Part model, mm, in its own coordinate system. A direction names the side the tool comes from. Round coordinates to 2 decimals unless told otherwise and drop trailing zeros. Order: outer loops, then holes, each group sorted by start corner. A loop starts at its lowest first (then second) coordinate and runs counter-clockwise, first axis right, second up. Notation, with made-up numbers: (-0.75, 68.25) -> (44.25, 68.25) arc R31 ccw to (44.25, 95.25) -> close; hole circle Ø8 at (-10, 57.5). An arc over 180 degrees is marked (long way). Use CSV: the item, a comma, the result in double quotes.
```python
from build123d import *

# Parameters (mm, degrees)
SKETCH_R     = 2.5
PAD_DEPTH    = 2
PAD001_DEPTH = 5
SKETCH002_R  = 2.5
PAD002_DEPTH = 30
PAD003_DEPTH = 5
SKETCH004_R  = 2.5
PAD004_DEPTH = 3


with BuildPart() as part:
    # Sketch → Pad (new body)
    with BuildSketch(Plane.XY):
        Circle(SKETCH_R)
    extrude(amount=PAD_DEPTH)

    # Sketch001 (on Face3 of Pad) → Pad001 (join)
    with BuildSketch(Plane.XY.offset(2)):
        Polygon((0.734523, 4.439648), (-3.477586, 2.85594), (-4.21211, -1.583708), (-0.734523, -4.439648), (3.477586, -2.85594), (4.21211, 1.583708), align=None)
    extrude(amount=PAD001_DEPTH)

    # Sketch002 (on Face5 of Pad001) → Pad002 (join)
    with BuildSketch(Plane.XY.offset(7)):
        Circle(SKETCH002_R)
    extrude(amount=PAD002_DEPTH)

    # Sketch003 (on Face12 of Pad002) → Pad003 (join)
    with BuildSketch(Plane.XY.offset(37)):
        Polygon((-1.455794, 4.258012), (-4.415443, 0.868251), (-2.959649, -3.38976), (1.455794, -4.258012), (4.415443, -0.868251), (2.959649, 3.38976), align=None)
    extrude(amount=PAD003_DEPTH)

    # Sketch004 (on Face5 of Pad003) → Pad004 (join)
    with BuildSketch(Plane.XY.offset(42)):
        Circle(SKETCH004_R)
    extrude(amount=PAD004_DEPTH)


solid = part.part
```
(1) Cut at C-C, the plane x = 2. Give the cut face in (y, z), then the cut area to 3 significant figures.
Reply:
outline,"(-3.63, 37) -> (-1.5, 37) -> (-1.5, 7) -> (-3.41, 7) -> (-3.41, 2) -> (-1.5, 2) -> (-1.5, 0) -> (1.5, 0) -> (1.5, 2) -> (3.4, 2) -> (3.4, 7) -> (1.5, 7) -> (1.5, 37) -> (3.58, 37) -> (3.58, 42) -> (1.5, 42) -> (1.5, 45) -> (-1.5, 45) -> (-1.5, 42) -> (-3.63, 42) -> close"
area,"175 mm2"
(2) Cut at D-D, the plane z = 15. Give the cut face in (x, y), then the cut area to 3 significant figures.
Reply:
outline,"circle Ø5 at (0, 0)"
area,"19.6 mm2"
(3) Drop flat-ended pins along their axis: P1, Ø1, axis at x = -1.5, y = 3, coming from the -Z side; P2, Ø4, axis at y = 2, z = 32, coming from the +X side; P3, Ø4, axis at x = -0.5, z = 29.5, coming from the -Y side. Give the stop position or say it passes through.
Reply:
P1,"z = 2"
P2,"x = 2.5"
P3,"y = -2.5"
(4) Which spindle directions (+Z, -Z, +X, -X, +Y, -Y) get a long thin tool onto all of the face, cutting with end or side? Do faces 1 (the face through (-3.7, -1.23, 39.47)), 2 (the face through (2, -2, 37)), 3 (the face through (2, -2, 42)). Say none if no direction does.
Reply:
face 1,"+Z, -X, -Y"
face 2,"none"
face 3,"+Z"
(5) Cut at B-B, the plane z = 40.5. Give the cut face in (x, y), then the cut area to 3 significant figures.
Reply:
outline,"(-4.42, 0.87) -> (-2.96, -3.39) -> (1.46, -4.26) -> (4.42, -0.87) -> (2.96, 3.39) -> (-1.46, 4.26) -> close"
area,"52.6 mm2"
(6) Probe probe 1 along Z at (x, y) = (-3.25, -1); probe 2 along X at (y, z) = (-0.75, 23); probe 3 along X at (y, z) = (-1.5, 15). List the from-to ranges inside material, lowest first. Write a range as [from, to].
Reply:
probe 1,"[2, 7], [37, 42]"
probe 2,"[-2.38, 2.38]"
probe 3,"[-2, 2]"
(7) Cut at A-A, the plane y = -2. Give the cut face in (x, z).
Reply:
outline,"(-3.71, 2) -> (-1.5, 2) -> (-1.5, 0) -> (1.5, 0) -> (1.5, 2) -> (3.62, 2) -> (3.62, 7) -> (1.5, 7) -> (1.5, 37) -> (3.43, 37) -> (3.43, 42) -> (1.5, 42) -> (1.5, 45) -> (-1.5, 45) -> (-1.5, 42) -> (-3.43, 42) -> (-3.43, 37) -> (-1.5, 37) -> (-1.5, 7) -> (-3.71, 7) -> close"
(8) Pull direction Z, two halves, no side cores. Call faces 4 (the face through (-2.91, 2.59, 39.47)), 5 (the face through (-2, -2, 7)), 6 (the face through (-2, -2, 2)), 7 (the face through (-0.54, -2.44, 21.79)): released by +Z, released by -Z, zero draft, split by the parting line, or undercut.
Reply:
face 4,"zero draft"
face 5,"undercut"
face 6,"released by -Z"
face 7,"undercut"
